Verification items for this drawing (mm, ordinates from the low corner). Give positions to 0.01 mm unless a question says otherwise; leave off trailing zeros. Loops run counter-clockwise (first coordinate to the right, second up) from the corner with the lowest first, then second, coordinate; pieces in that order, holes last. Notation, with made-up numbers: (-33, 59.5) -> (-28, 59.5) arc R6 ccw to (-28, 67.5) -> close; hole circle Ø9 at (9.5, 10.5). An arc over 180 degrees is marked (long way). Write each question's results on one line, items separated by ' | '. Start each with the question number.
Item 1: Cross-section at D-D on y = 19.5. Enter the section's corners in (x, z).
Item 2: Scan lines: line 1 along Y through (x, z) = (5, 3); line 2 along X through (y, z) = (19, 8); line 3 along X through (y, z) = (27, 6.5). Record each from-to range of solid material in increasing order.
Item 3: Gauge pin test, flat ends, axial feed: pin 1 Ø10 at (x, y) = (72.5, 28.5) entering from +Z; pin 2 Ø2.5 at (x, z) = (72.5, 8) entering from +Y; pin 3 Ø1.5 at (x, z) = (52.5, 5.5) entering from -Y. Record the tip position at first contact, or that the pin passes through.
Item 4: Cross-section at A-A on x = 115. Enter the section's corners in (y, z), then the cut area to 3 significant figures.
Item 5: Cross-section at C-C on x = 23. Enter the section's corners in (y, z), then the cut area to 3 significant figures.
Item 6: Cross-section at B-B on y = 11. Enter the section's corners in (x, z), then the cut area to 3 significant figures.
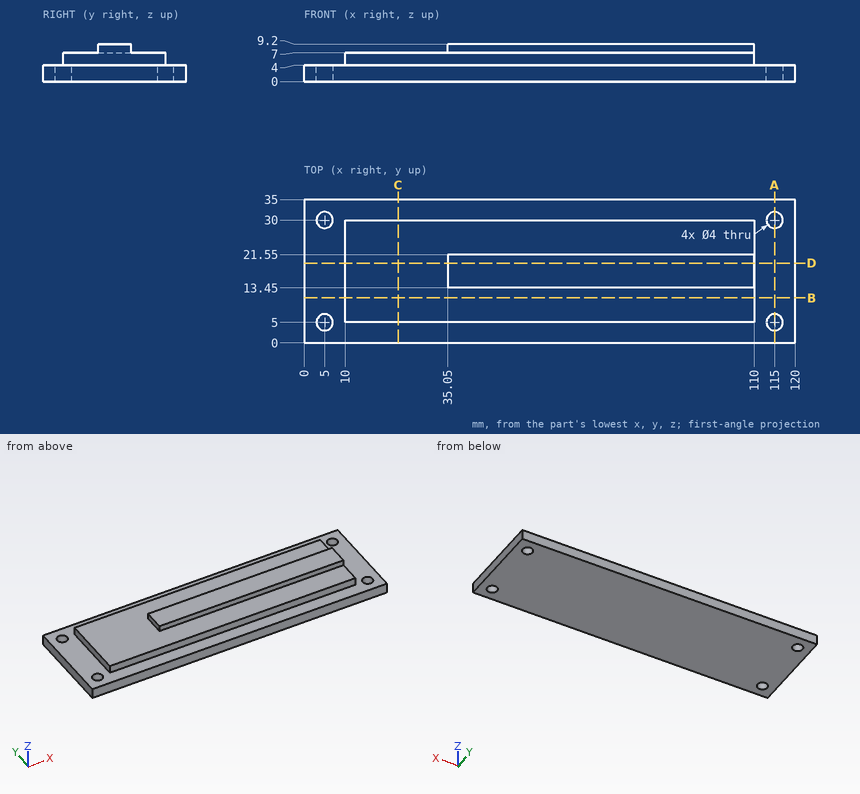
Answer sheet:
1) outline: (0, 0) -> (120, 0) -> (120, 4) -> (110, 4) -> (110, 9.2) -> (35.05, 9.2) -> (35.05, 7) -> (10, 7) -> (10, 4) -> (0, 4) -> close
2) line 1: y = 0 to 3, 7 to 28, 32 to 35 | line 2: x = 35.05 to 110 | line 3: x = 10 to 110
3) pin 1: stops at z = 7 | pin 2: stops at y = 30 | pin 3: stops at y = 5
4) outline: (0, 0) -> (3, 0) -> (3, 4) -> (0, 4) -> close; (7, 0) -> (28, 0) -> (28, 4) -> (7, 4) -> close; (32, 0) -> (35, 0) -> (35, 4) -> (32, 4) -> close | area: 108 mm²
5) outline: (0, 0) -> (35, 0) -> (35, 4) -> (30, 4) -> (30, 7) -> (5, 7) -> (5, 4) -> (0, 4) -> close | area: 215 mm²
6) outline: (0, 0) -> (120, 0) -> (120, 4) -> (110, 4) -> (110, 7) -> (10, 7) -> (10, 4) -> (0, 4) -> close | area: 780 mm²
